Geometry: see drawing. Coordinates: mm, zero at the bounding-box minimum. Give positions to 0.01 mm unless a question says otherwise; leave off trailing zeros. Write each loop counter-clockwise with the first axis right and the second up, starting at its lowest first coordinate (ties: lowest second). Pieces come first, ordered by that corner, then holes. Notation, with made-up numbers: (-12.5, 37.25) - (43.5, 37.25) arc R18 ccw to (43.5, 69.25) - close; hole circle Ø4 at (30, -11.75). An arc over 180 degrees is marked (long way). Use a Markdown table: item, result. Add a question column.
1. Material intervals for probe 1 along Z at (x, y) = (6.75, 0.15); probe 2 along X at (y, z) = (0.1, 2.25) (1 decimal); probe 3 along X at (y, z) = (0.2, 3.75) (1 decimal), sorted ascending.
2. Section query D-D, the plane x = 1.25. Return loops of the section in (y, z).
3. Section query A-A, the plane x = 3.5. Return loops of the section in (y, z).
4. Section query B-B, the plane y = 0.1. Count the separate pieces of the cut face and the enclosed holes in it.
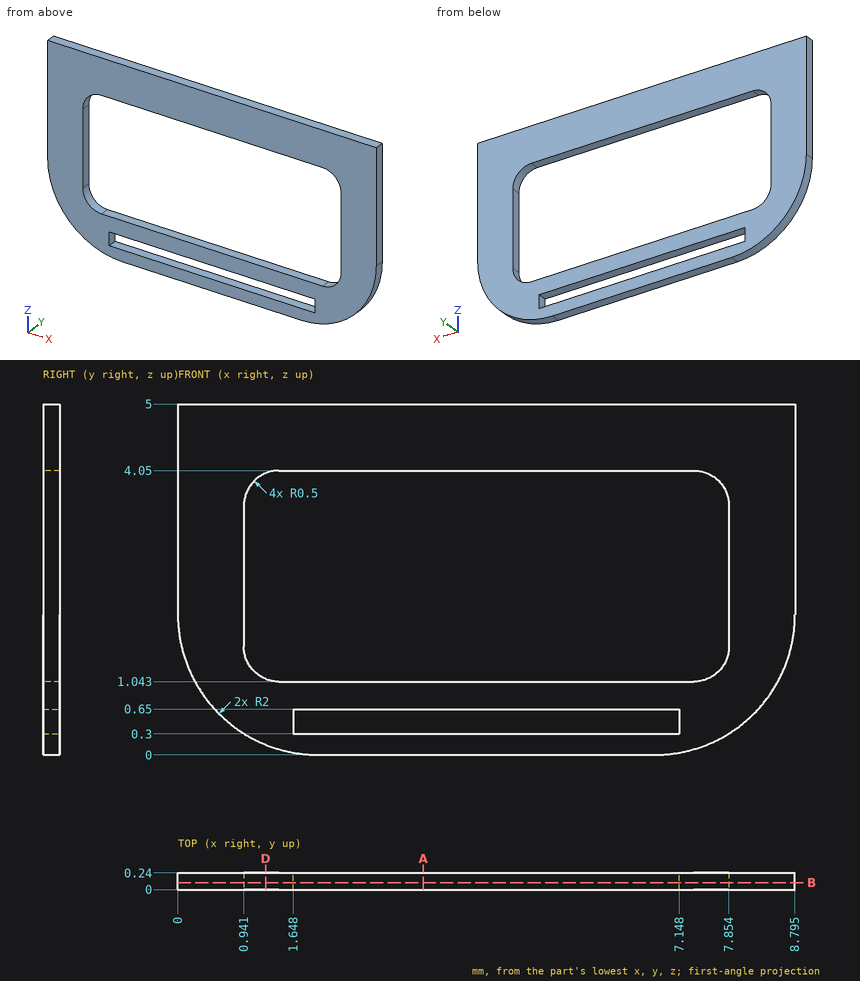
Result sheet:
| question | item | result |
|---|---|---|
| 1 | probe 1 | z = 0 to 0.3, 0.65 to 1.04, 4.05 to 5 |
| 1 | probe 2 | x = 0 to 0.9, 7.9 to 8.8 |
| 1 | probe 3 | x = 0 to 1, 7.8 to 8.8 |
| 2 | outline | (0, 0.15) - (0.24, 0.15) - (0.24, 1.08) - (0, 1.08) - close; (0, 4.01) - (0.24, 4.01) - (0.24, 5) - (0, 5) - close |
| 3 | outline | (0, 0) - (0.24, 0) - (0.24, 0.3) - (0, 0.3) - close; (0, 0.65) - (0.24, 0.65) - (0.24, 1.04) - (0, 1.04) - close; (0, 4.05) - (0.24, 4.05) - (0.24, 5) - (0, 5) - close |
| 4 | separate pieces | 1 |
| 4 | enclosed holes | 2 |
